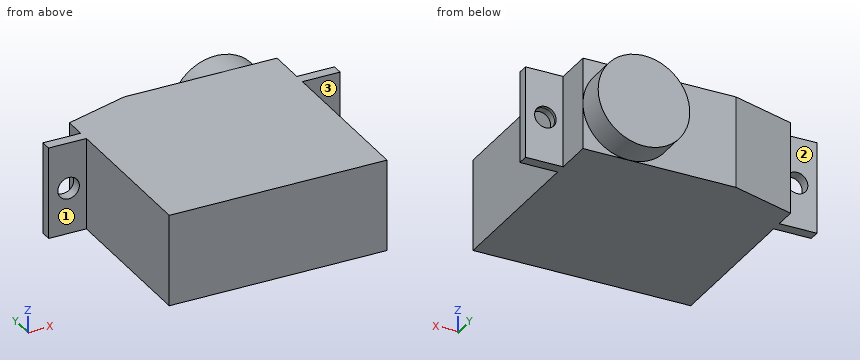
from build123d import *

# Parameters (mm, degrees)
BOSS_EXTRUDE1_DEPTH     = 8.5
SKETCH2_R               = 4.25
BOSS_EXTRUDE2_DEPTH     = 2.7
SKETCH3_R               = 1
CUT_EXTRUDE1_DEPTH      = 7.5
CUT_EXTRUDE1_DEPTH_BACK = 16.7


with BuildPart() as part:
    # Sketch1 → Boss-Extrude1 (new body)
    with BuildSketch(Plane.XY):
        Polygon((0, 0), (-20.2, 0), (-20.2, 14.7), (-23.7, 14.7), (-23.7, 15.7), (-20.2, 15.7), (-20.2, 17.7), (-14.2, 19.5), (0, 19.5), (0, 16), (3.5, 16), (3.5, 15), (0, 15), align=None)
    extrude(amount=BOSS_EXTRUDE1_DEPTH)

    # Sketch2 → Boss-Extrude2 (add)
    with BuildSketch(Plane(origin=(0, 19.5, 0), x_dir=(1, 0, 0), z_dir=(0, 1, 0))):
        with Locations((-4.25, -4.25)):
            Circle(SKETCH2_R)
    extrude(amount=BOSS_EXTRUDE2_DEPTH)

    # Sketch3 → Cut-Extrude1 (cut, two sides)
    with BuildSketch(Plane(origin=(0, 15.7, 0), x_dir=(1, 0, 0), z_dir=(0, 1, 0))) as cut_extrude1_sk:
        with Locations((-21.85, -4.25)):
            Circle(SKETCH3_R)
        with Locations((1.65, -4.25)):
            Circle(SKETCH3_R)
    extrude(amount=CUT_EXTRUDE1_DEPTH, mode=Mode.SUBTRACT)
    extrude(cut_extrude1_sk.sketch, amount=-CUT_EXTRUDE1_DEPTH_BACK, mode=Mode.SUBTRACT)


solid = part.part
Geometry: final body of the model. Coordinates: model frame, mm. Face numbers are marked on the shaded views. A direction names the side the tool comes from. Give positions to 0.01 mm unless a question says otherwise; leave off trailing zeros. Write each loop counter-clockwise with the first axis right and the second up, starting at its lowest first coordinate (ties: lowest second). Pieces come first, ordered by that corner, then holes. Notation, with made-up numbers: (77, 88.25) -> (104, 88.25) arc R20 ccw to (104, 126.25) -> close; hole circle Ø4 at (14, 23). An arc over 180 degrees is marked (long way). Answer in a Markdown table with one row per item.
(1) Ray query, line 1 along X through (y, z) = (15.25, 4.25); line 2 along X through (y, z) = (15.95, 4.25); line 3 along Z through (x, y) = (1.65, 15.8). Return the intervals inside material, ascending. Write a range as [from, to].
Answers below:
| item | result |
|---|---|
| line 1 | [-23.7, -22.85], [-20.85, 0.65], [2.65, 3.5] |
| line 2 | [-20.2, 0.65], [2.65, 3.5] |
| line 3 | [0, 3.25], [5.25, 8.5] |
(2) Section query D-D on x = -13.25. Return loops of the section in (y, z), then the cut area to 3 significant figures.
Answers below:
| item | result |
|---|---|
| outline | (0, 0) -> (19.5, 0) -> (19.5, 8.5) -> (0, 8.5) -> close |
| area | 166 mm^2 |
(3) Set-up query: the marked faces 1, 2 and 3. Return all of +Z, -Z, +X, -X, +Y, -Y with unobstructed straight access to the full face (end or side cutting, diameter ignored); none if empty.
Answers below:
| item | result |
|---|---|
| face 1 | +Z, -Z, -X, -Y |
| face 2 | +Z, -Z, -X, +Y |
| face 3 | +Z, -Z, +X, -Y |
(4) Section query A-A on x = -21.85. Return loops of the section in (y, z).
Answers below:
| item | result |
|---|---|
| outline | (14.7, 0) -> (15.7, 0) -> (15.7, 3.25) -> (14.7, 3.25) -> close; (14.7, 5.25) -> (15.7, 5.25) -> (15.7, 8.5) -> (14.7, 8.5) -> close |
(5) Section query B-B on z = 6.25. Return loops of the section in (x, y), then the cut area to 3 significant figures.
Answers below:
| item | result |
|---|---|
| outline | (-23.7, 14.7) -> (-20.2, 14.7) -> (-20.2, 0) -> (0, 0) -> (0, 15) -> (3.5, 15) -> (3.5, 16) -> (0, 16) -> (0, 19.5) -> (-0.5, 19.5) -> (-0.5, 22.2) -> (-8, 22.2) -> (-8, 19.5) -> (-14.2, 19.5) -> (-20.2, 17.7) -> (-20.2, 15.7) -> (-23.7, 15.7) -> close |
| area | 416 mm^2 |
(6) Section query C-C on y = 11. Return loops of the section in (x, z), then the cut area to 3 significant figures.
Answers below:
| item | result |
|---|---|
| outline | (-20.2, 0) -> (0, 0) -> (0, 8.5) -> (-20.2, 8.5) -> close |
| area | 172 mm^2 |
(7) Pin query (flat end, axial travel): pin 1 (1.2 mm diameter, centred on x = 1.65, z = 4.25, fed in from +Y); pin 2 (1 mm diameter, centred on y = 18, z = 5.5, fed in from +X); pin 3 (3 mm diameter, centred on y = 11, z = 1, fed in from -X); pin 4 (4 mm diameter, centred on x = -22.5, z = 4.5, fed in from +Y). Return the tip coordinate at first contact, or that it passes through.
Answers below:
| item | result |
|---|---|
| pin 1 | through |
| pin 2 | x = 0 |
| pin 3 | x = -20.2 |
| pin 4 | y = 15.7 |
